Could you check a few things on this model? Use its own coordinates, in mm. A direction names the side the tool comes from. Coordinates: 2 decimals unless noted, no trailing zeros. Order: outer loops, then holes, each group sorted by start corner. A loop starts at its lowest first (then second) coordinate and runs counter-clockwise, first axis right, second up. Notation, with made-up numbers: (63, -6.5) -> (80, -6.5) arc R12 ccw to (80, 12.5) -> close; hole circle Ø5 at (-23.5, -25). An arc over 180 degrees is marked (long way). Use a Markdown table: item, result. Add a question column.
1) Will these pins go through, and if not, where does the flat tip stop? pin 1 Ø2 at (x, z) = (19, -9.5) entering from +Y; pin 2 Ø5 at (x, y) = (-20, 4) entering from -Z; pin 3 Ø6 at (y, z) = (7, 4.5) entering from +X; pin 4 Ø3 at (y, z) = (2, 2.5) entering from -X.
2) If we section it at D-D (x = 4.5): Write out the boundary of the cut face in (y, z).
3) If we section it at A-A (x = -34): Write out the boundary of the cut face in (y, z).
4) If I drill on L1, parallel to Z at x = -22.5, y = 7; L2, parallel to Y at x = -40, z = -6.7; L3, parallel to Z at x = -1.5, y = 7.75, over which ranges is the centre line in solid material (lowest first)? Write a range as [from, to].
5) Which directions (+Z, -Z, +X, -X, +Y, -Y) give clear straight access to the entire face, cutting with the end or side of a thin tool? Please do faces 3 (the flat face through (-33, 5, 5)), 4 (the flat face through (-26, 5, -10)), 5 (the flat face through (10.56, 5.07, 18.15)).
6) If we section it at B-B (y = 9): Write out the boundary of the cut face in (x, z).
7) Thinking about a two-plate mould opening in Y: for faces 1 (the flat face through (15.97, 4.93, -42.74)), 2 (the cylindrical face through (27.06, 4.09, 31.94)), which applies, +Y half, -Y half, draft (parallel to the pull), parting line (faces both ways), or undercut?
8) If we section it at C-C (z = 24.5): Write out the boundary of the cut face in (x, y), plus the area to 3 significant figures.
```python
from build123d import *

# Parameters (mm, degrees)
SKETCH1_W          = 45
SKETCH1_H          = 10
MAIN_DEPTH         = 10
CUT_EXTRUDE1_START = -21
SKETCH2_R          = 1.5
CUT_EXTRUDE1_DEPTH = 22
SKETCH4_W          = 24
SKETCH4_H          = 10
CUT_EXTRUDE3_DEPTH = 11
CIRPATTERN1_COUNT  = 3
SKETCH3_R          = 3
CUT_EXTRUDE2_DEPTH = 11


with BuildPart() as part:
    # Sketch1 → Main (new body, symmetric)
    with BuildSketch(Plane.XY):
        with Locations((-22.5, 5)):
            Rectangle(SKETCH1_W, SKETCH1_H)
    main = extrude(amount=MAIN_DEPTH, both=True)

    # Sketch2 → Cut-Extrude1 (cut)
    with BuildSketch(Plane.XY.offset(10).offset(CUT_EXTRUDE1_START)):
        with Locations((-40, 5)):
            Circle(SKETCH2_R)
    cut_extrude1 = extrude(amount=CUT_EXTRUDE1_DEPTH, mode=Mode.SUBTRACT)

    # Sketch4 → Cut-Extrude3 (cut, through all)
    with BuildSketch(Plane(origin=(0, 10, 0), x_dir=(1, 0, 0), z_dir=(0, 1, 0))):
        with Locations((-33, 0)):
            Rectangle(SKETCH4_W, SKETCH4_H)
    cut_extrude3 = extrude(amount=-CUT_EXTRUDE3_DEPTH, mode=Mode.SUBTRACT)

    # CirPattern1: Main, Cut-Extrude1, Cut-Extrude3 ×3 about axis
    cirpattern1_axis = Axis((0, 0, 0), (0, 1, 0))
    for i in range(1, CIRPATTERN1_COUNT):
        add(main.rotate(cirpattern1_axis, i * 360 / CIRPATTERN1_COUNT))
        add(cut_extrude1.rotate(cirpattern1_axis, i * 360 / CIRPATTERN1_COUNT), mode=Mode.SUBTRACT)
        add(cut_extrude3.rotate(cirpattern1_axis, i * 360 / CIRPATTERN1_COUNT), mode=Mode.SUBTRACT)

    # Sketch3 → Cut-Extrude2 (cut, through all)
    with BuildSketch(Plane(origin=(0, 10, 0), x_dir=(1, 0, 0), z_dir=(0, 1, 0))):
        Circle(SKETCH3_R)
    extrude(amount=-CUT_EXTRUDE2_DEPTH, mode=Mode.SUBTRACT)


solid = part.part
```
Answer sheet:
| question | item | result |
|---|---|---|
| 1 | pin 1 | through |
| 1 | pin 2 | z = -10 |
| 1 | pin 3 | x = 15.88 |
| 1 | pin 4 | x = -21 |
| 2 | outline | (0, -27.79) -> (10, -27.79) -> (10, 27.79) -> (0, 27.79) -> close |
| 3 | outline | (0, -10) -> (10, -10) -> (10, -5) -> (0, -5) -> close; (0, 5) -> (10, 5) -> (10, 10) -> (0, 10) -> close |
| 4 | L1 | [-10, -5], [5, 10] |
| 4 | L2 | [0, 3.5], [6.5, 10] |
| 4 | L3 | [-17.4, -2.6], [2.6, 17.4] |
| 5 | face 3 | -X, +Y, -Y |
| 5 | face 4 | -Z, -X, +Y, -Y |
| 5 | face 5 | +Y, -Y |
| 6 | outline | (-45, -10) -> (-5.77, -10) -> (13.84, -43.97) -> (18.17, -41.47) -> (6.17, -20.69) -> (14.83, -15.69) -> (26.83, -36.47) -> (31.16, -33.97) -> (11.55, 0) -> (31.16, 33.97) -> (26.83, 36.47) -> (14.83, 15.69) -> (6.17, 20.69) -> (18.17, 41.47) -> (13.84, 43.97) -> (-5.77, 10) -> (-45, 10) -> (-45, 5) -> (-21, 5) -> (-21, -5) -> (-45, -5) -> close; hole circle Ø6 at (0, 0) |
| 7 | face 1 | draft |
| 7 | face 2 | undercut |
| 8 | outline | (2.6, 0) -> (8.37, 0) -> (8.37, 10) -> (2.6, 10) -> close; (19.92, 0) -> (25.69, 0) -> (25.69, 10) -> (19.92, 10) -> close |
| 8 | area | 115 mm2 |
